Part model, mm, in its own coordinate system. A direction names the side the tool comes from. Coordinates: 2 decimals unless noted, no trailing zeros.
1) Cut at A-A (z = 1.6). Give the number of separate pieces and of enclosed holes in the cut face, and give its area (3 significant figures).
2) Wall check: L1, parallel to X at y = 44.5, z = 0.4; L2, parallel to X at y = 82.55, z = 1.95 (3 decimals); L3, parallel to X at y = -55, z = 1.7. Give the ranges that are in metal, low to high.
3) Tool access for faces 1 (the flat face through (-5, 45, 3.81)), 2 (the cylindrical face through (0.08, -10.16, 1.88)): list every direction of +Z, -Z, +X, -X, +Y, -Y with a clear straight run to the whole face (end or side of a thin tool).
4) Mould opens along X. For faces 3 (the cylindrical face through (-1.707, 79.873, 1.878)), 4 (the flat face through (-5, 45, 0)) say: +X half, -X half, draft (parallel to the pull), parting line (faces both ways), or undercut.
5) Pin check, flat tip, straight feed: pin 1 Ø5 at (x, y) = (0, -31.75) entering from +Z. Stop position of the tip, or through.
```python
from build123d import *

# Parameters (mm, degrees)
SKETCH1_R          = 3.175
MAIN_EXTRUDE_DEPTH = 3.81


with BuildPart() as part:
    # Sketch1 → Main extrude (new body)
    with BuildSketch(Plane.XY):
        with BuildLine():
            add(Edge.make_bspline(
                [(0, 140.978035645), (3.918482074, 131.156065717), (8.169378172, 106.05556313), (10.242574642, 81.433345605), (11.145665597, 45.040166844), (8.163737965, -35.508846412), (0, -109.12531842)],
                knots=[0.045526815, 0.045526815, 0.045526815, 0.20753057, 0.315533073, 0.423535576, 0.585539331, 0.909546841, 0.909546841, 0.909546841], degree=2))
            add(Edge.make_bspline(
                [(0, -109.12531842), (-8.163737965, -35.508846412), (-11.145665597, 45.040166844), (-10.242574642, 81.433345605), (-8.169378172, 106.05556313), (-3.918482074, 131.156065717), (0, 140.978035645)],
                knots=[0.045526815, 0.045526815, 0.045526815, 0.369534325, 0.53153808, 0.639540583, 0.747543086, 0.909546841, 0.909546841, 0.909546841], degree=2))
        make_face()
        with Locations(Location((0, 82.55, 0), (0, 0, 180))):
            Circle(SKETCH1_R, mode=Mode.SUBTRACT)
        with Locations(Location((0, -31.75, 0), (0, 0, 180))):
            Circle(SKETCH1_R, mode=Mode.SUBTRACT)
        with BuildLine():
            Line((3.81, 57.15), (3.81, -6.35))
            ThreePointArc((3.81, -6.35), (0, -10.16), (-3.81, -6.35))
            Line((-3.81, -6.35), (-3.81, 57.15))
            ThreePointArc((-3.81, 57.15), (0, 60.96), (3.81, 57.15))
        make_face(mode=Mode.SUBTRACT)
    extrude(amount=MAIN_EXTRUDE_DEPTH)


solid = part.part
```
Geometry check:
1. separate pieces: 1
1. enclosed holes: 3
1. area: 3,010 mm2
2. L1: x = -10.77 to -3.81, 3.81 to 10.77
2. L2: x = -9.983 to -3.175, 3.175 to 9.983
2. L3: x = -5.41 to 5.41
3. face 1: +Z, +X, -X, +Y, -Y
3. face 2: +Z, -Z
4. face 3: undercut
4. face 4: draft
5. pin 1: passes through
